Could you check a few things on this model? Use its own coordinates, in mm. A direction names the side the tool comes from. Coordinates: 2 decimals unless noted, no trailing zeros. Order: outer loops, then holes, each group sorted by start corner. A loop starts at its lowest first (then second) coordinate and runs counter-clockwise, first axis right, second up. Notation, with made-up numbers: (86.25, -19) - (102.25, -19) arc R15 cw to (102.25, -10) - close; hole circle Ø8 at (55, 82.5). An arc over 180 degrees is marked (long way). Answer as a JSON object with one key per item and string values. Group by question number.
(1) Please list where these lines run through material, in increasing order: probe 1 along Z at (x, y) = (4.75, 0); probe 2 along Z at (x, y) = (0.5, 0).
(2) Imagine slicing it at D-D, the plane x = 6.25. Write out the boundary of the cut face in (y, z), and give its area (3 significant figures).
(3) Imagine slicing it at C-C, the plane y = 0. Write out the boundary of the cut face in (x, z), and give its area (3 significant figures).
(4) Imagine slicing it at B-B, the plane x = -2.75. Write out the boundary of the cut face in (y, z), and give its area (3 significant figures).
(5) Will these pins go through, and if not, where does the flat tip stop? P1, Ø7, axis at y = -1, z = 2.5, coming from the +X side; P2, Ø2, axis at x = 1.5, z = 4, coming from the -Y side; P3, Ø2, axis at y = -3, z = 0, coming from the -X side; P4, Ø0.6, axis at y = 4, z = 0, coming from the -X side.
(6) We'd pull the mould along X, two halves only. Please class faces 1 (the flat face through (0, 4, 4)), 2 (the flat face through (-2.28, -6.09, -3.45)), 3 (the flat face through (-4.6, 4, 0)): pulls with the +X half, pulls with the -X half, needs draft (parallel to the pull), parting line crosses it, or undercut.
(7) Imagine slicing it at A-A, the plane x = 8.25. Write out the boundary of the cut face in (y, z).
(8) Which directions (+Z, -Z, +X, -X, +Y, -Y) give clear straight access to the entire face, cutting with the end or side of a thin tool? Please do faces 4 (the flat face through (-2.277, -6.034, 3.549)), 5 (the cylindrical face through (-4.8, -0.01, -2.46)).
from build123d import *

# Parameters (mm, degrees)
SKETCH2_W          = 10.6
SKETCH2_H          = 4.3
SKETCH3_W          = 40
SKETCH3_H          = 40
CUT_EXTRUDE1_DEPTH = 6.5
CUT_EXTRUDE2_DEPTH = 2.29
SKETCH5_W          = 1.9
SKETCH5_H          = 10.8
CUT_EXTRUDE3_DEPTH = 1.4


with BuildPart() as part:
    # Sketch1 → Revolve1 (revolve)
    with BuildSketch(Plane.XY):
        with BuildLine():
            Line((-2.490737563, 10), (0, 10))
            Line((0, 10), (0, 5.3865))
            Line((0, 5.3865), (0.6365, 5.3865))
            Line((0.6365, 5.3865), (1.25, 6))
            Line((1.25, 6), (7.15, 6))
            Line((7.15, 6), (8, 5.15))
            Line((8, 5.15), (9, 5.15))
            Line((9, 5.15), (9, 0))
            Line((9, 0), (-6, 0))
            ThreePointArc((-6, 0), (-5.206361598, 5.133599494), (-2.899547792, 9.787878788))
            ThreePointArc((-2.899547792, 9.787878788), (-2.721020656, 9.943812682), (-2.490737563, 10))
        make_face()
    revolve(axis=Axis((9, 0, 0), (-1, 0, 0)))

    # Sketch2 → Cut-Revolve1 (revolve, cut)
    with BuildSketch(Plane.XY):
        with Locations((3.7, 2.15)):
            Rectangle(SKETCH2_W, SKETCH2_H)
    revolve(axis=Axis((9, 0, 0), (-1, 0, 0)), mode=Mode.SUBTRACT)

    # Sketch3 → Cut-Extrude1 (cut)
    with BuildSketch(Plane(origin=(-6, 0, 0), x_dir=(0, 0, -1), z_dir=(1, 0, 0))):
        Rectangle(SKETCH3_W, SKETCH3_H)
        Polygon((-7, -4.041451884), (0, -8.082903769), (7, -4.041451884), (7, 4.041451884), (0, 8.082903769), (-7, 4.041451884), align=None, mode=Mode.SUBTRACT)
    extrude(amount=CUT_EXTRUDE1_DEPTH, mode=Mode.SUBTRACT)

    # Sketch4 → Cut-Extrude2 (cut)
    with BuildSketch(Plane(origin=(-6, 0, 0), x_dir=(0, 0, -1), z_dir=(1, 0, 0))):
        with BuildLine():
            Line((-2.189430305, -0.450302912), (-1.45357474, -0.841564257))
            Line((-1.45357474, -0.841564257), (-0.852063671, -0.852063671))
            Line((-0.852063671, -0.852063671), (-0.841564257, -1.45357474))
            Line((-0.841564257, -1.45357474), (-0.450302912, -2.189430305))
            ThreePointArc((-0.450302912, -2.189430305), (0, -2.459999131), (0.450302912, -2.189430305))
            Line((0.450302912, -2.189430305), (0.841564257, -1.45357474))
            Line((0.841564257, -1.45357474), (0.852063671, -0.852063671))
            Line((0.852063671, -0.852063671), (1.45357474, -0.841564257))
            Line((1.45357474, -0.841564257), (2.189430305, -0.450302912))
            ThreePointArc((2.189430305, -0.450302912), (2.459999131, 0), (2.189430305, 0.450302912))
            Line((2.189430305, 0.450302912), (1.45357474, 0.841564257))
            Line((1.45357474, 0.841564257), (0.852063671, 0.852063671))
            Line((0.852063671, 0.852063671), (0.841564257, 1.45357474))
            Line((0.841564257, 1.45357474), (0.450302912, 2.189430305))
            ThreePointArc((0.450302912, 2.189430305), (0, 2.459999131), (-0.450302912, 2.189430305))
            Line((-0.450302912, 2.189430305), (-0.841564257, 1.45357474))
            Line((-0.841564257, 1.45357474), (-0.852063671, 0.852063671))
            Line((-0.852063671, 0.852063671), (-1.45357474, 0.841564257))
            Line((-1.45357474, 0.841564257), (-2.189430305, 0.450302912))
            ThreePointArc((-2.189430305, 0.450302912), (-2.459999131, 0), (-2.189430305, -0.450302912))
        make_face()
    extrude(amount=CUT_EXTRUDE2_DEPTH, mode=Mode.SUBTRACT)

    # Sketch5 → Cut-Extrude3 (cut)
    with BuildSketch(Plane(origin=(-6, 0, 0), x_dir=(0, 0, -1), z_dir=(1, 0, 0))):
        Rectangle(SKETCH5_W, SKETCH5_H)
    extrude(amount=CUT_EXTRUDE3_DEPTH, mode=Mode.SUBTRACT)


solid = part.part
Result set:
{
 "1": {"probe 1": "z = -6 to -4.3, 4.3 to 6", "probe 2": "z = -5.39 to -4.3, 4.3 to 5.39"},
 "2": {"outline": "circle Ø12 at (0, 0); hole circle Ø8.6 at (0, 0)", "area": "55.0 mm^2"},
 "3": {"outline": "(-5.82, -2.46) arc R17 ccw to (-4.49, -7) - (0, -7) - (0, -5.39) - (0.64, -5.39) - (1.25, -6) - (7.15, -6) - (8, -5.15) - (9, -5.15) - (9, -4.3) - (-1.6, -4.3) - (-1.6, 4.3) - (9, 4.3) - (9, 5.15) - (8, 5.15) - (7.15, 6) - (1.25, 6) - (0.64, 5.39) - (0, 5.39) - (0, 7) - (-4.49, 7) arc R17 ccw to (-5.82, 2.46) - (-3.71, 2.46) - (-3.71, -2.46) - close", "area": "79.4 mm^2"},
 "4": {"outline": "(-8.08, 0) - (-4.04, -7) - (4.04, -7) - (8.08, 0) - (4.04, 7) - (-4.04, 7) - close", "area": "170 mm^2"},
 "5": {"P1": "stops at x = 9", "P2": "stops at y = -5.2", "P3": "stops at x = -5.76", "P4": "stops at x = -4.6"},
 "6": {"face 1": "undercut", "face 2": "needs draft", "face 3": "pulls with the -X half"},
 "7": {"outline": "circle Ø10.3 at (0, 0); hole circle Ø8.6 at (0, 0)"},
 "8": {"face 4": "+Z, +X, -X, -Y", "face 5": "-X"}
}
